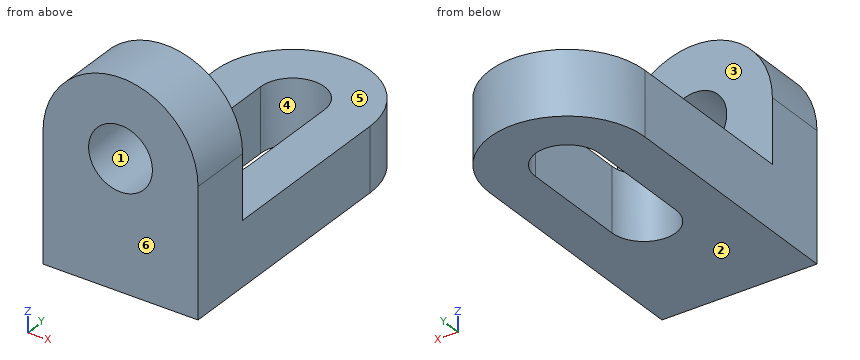
```python
from build123d import *

# Parameters (mm, degrees)
F1_DEPTH = 14
F2_R     = 7
F3_DEPTH = 14


with BuildPart() as f1:
    # F0 (on Top) → F1 (new body)
    with BuildSketch(Plane.XY):
        with BuildLine():
            Line((0, 54), (0, 0))
            Line((0, 0), (34, 0))
            Line((34, 0), (34, 54))
            ThreePointArc((34, 54), (17, 71), (0, 54))
        make_face()
        with BuildLine():
            ThreePointArc((10, 54), (17, 61), (24, 54))
            Line((24, 54), (24, 30))
            ThreePointArc((24, 30), (17, 23), (10, 30))
            Line((10, 30), (10, 54))
        make_face(mode=Mode.SUBTRACT)
    extrude(amount=F1_DEPTH)

    # F2 (on face) → F3 (join)
    with BuildSketch(Plane.XZ):
        with BuildLine():
            Line((0, 28), (0, 14))
            Line((0, 14), (34, 14))
            Line((34, 14), (34, 28))
            ThreePointArc((34, 28), (17, 45), (0, 28))
        make_face()
        with Locations((17, 28)):
            Circle(F2_R, mode=Mode.SUBTRACT)
    extrude(amount=-F3_DEPTH)


solid = f1.part
```
Here's how the part is built. I have some questions about the finished solid (model axes, mm). Face numbers are marked on the shaded views. A direction names the side the tool comes from. Coordinates: 2 decimals unless noted, no trailing zeros. Order: outer loops, then holes, each group sorted by start corner. A loop starts at its lowest first (then second) coordinate and runs counter-clockwise, first axis right, second up. Notation, with made-up numbers: (75.25, -33) - (90.25, -33) arc R4 ccw to (90.25, -27) - close; hole circle Ø3 at (16, -31.75). An arc over 180 degrees is marked (long way). One line per question, with ' | ' between items. Start each with the question number.
1. If we section it at C-C (z = 29.5): Write out the boundary of the cut face in (x, y).
2. I'm going to push flat-ended pins straight in: pin 1 Ø8.5 at (x, z) = (17, 28) entering from +Y; pin 2 Ø10 at (y, z) = (8, 8) entering from -X; pin 3 Ø6 at (x, z) = (23, 11.5) entering from +Y; pin 4 Ø1 at (y, z) = (62, 11) entering from +X. Where does each tip first touch, or does it pass through?
3. If we section it at A-A (y = 53): Write out the boundary of the cut face in (x, z), and give its area (3 significant figures).
4. Please list where these lines run through material, in increasing order: line 1 along Z through (x, y) = (17, 8.25); line 2 along Y through (x, z) = (11.5, 33). Write a range as [from, to].
5. Which directions (+Z, -Z, +X, -X, +Y, -Y) give clear straight access to the entire face, cutting with the end or side of a thin tool? Please do the marked faces 4, 5 and 6.
6. If we section it at D-D (z = 7.5): Write out the boundary of the cut face in (x, y), and give its area (3 significant figures).
7. If we section it at B-B (x = 17): Write out the boundary of the cut face in (y, z), and give its area (3 significant figures).
8. If we mould it in two halves opening along Z, with no side actions, what happens to the marked faces 1, 2 and 3? For each: released by +Z, released by -Z, zero draft, split by the parting line, or undercut.
Model answer:
1) outline: (0.07, 0) - (10.16, 0) - (10.16, 14) - (0.07, 14) - close; (23.84, 0) - (33.93, 0) - (33.93, 14) - (23.84, 14) - close
2) pin 1: passes through | pin 2: stops at x = 0 | pin 3: stops at y = 70.73 | pin 4: stops at x = 32.26
3) outline: (0, 0) - (10, 0) - (10, 14) - (0, 14) - close; (24, 0) - (34, 0) - (34, 14) - (24, 14) - close | area: 280 mm²
4) line 1: z = [0, 21], [35, 45] | line 2: y = [0, 14]
5) face 4: +Z, -Z | face 5: +Z, +X, -X, +Y | face 6: +Z, -Z, +X, -X, -Y
6) outline: (0, 0) - (34, 0) - (34, 54) arc R17 ccw to (0, 54) - close; hole (10, 30) arc R7 ccw to (24, 30) - (24, 54) arc R7 ccw to (10, 54) - close | area: 1,800 mm²
7) outline: (0, 0) - (23, 0) - (23, 14) - (14, 14) - (14, 21) - (0, 21) - close; (0, 35) - (14, 35) - (14, 45) - (0, 45) - close; (61, 0) - (71, 0) - (71, 14) - (61, 14) - close | area: 700 mm²
8) face 1: undercut | face 2: released by -Z | face 3: zero draft
